Design review of the part built by this model. Coordinates are the model's own, in mm. A direction names the side the tool comes from. Coordinates: 2 decimals unless noted, no trailing zeros. Loops run counter-clockwise (first coordinate to the right, second up) from the corner with the lowest first, then second, coordinate; pieces in that order, holes last. Notation, with made-up numbers: (-15.5, -31) -> (43.5, -31) arc R21 ccw to (43.5, -19) -> close; hole circle Ø2 at (8, -4.75). An arc over 180 degrees is marked (long way). Answer as a JSON object with one key per item and string values.
Autodesk Inventor part; units mm, degrees
ref_plane "Work Plane1" through (-5.715, 0, 0) normal (1, 0, 0) x (0, 1, 0)
ref_plane "Work Plane2" through (-5.715, 0, 0) normal (1, 0, 0) x (0, 1, 0)
ref_plane "XZ Plane" through (0, 0, 0) normal (0, 1, 0) x (-1, 0, 0)
sketch "Sketch1" plane through (0, 0, 0) normal (0, 1, 0) x (-1, 0, 0)
  circle A0 centre (0, 0) radius 4.318
  circle A1 centre (0, 0) radius 5.715
  dimension "d0" = 8.636
  dimension "d1" = 11.43
extrude "Extrusion1" add sketch "Sketch1" along normal blind 3.302
sketch "Sketch2" plane through (0, 0, 0) normal (0, -1, 0) x (1, 0, 0)
  circle A0 centre (0, 0) radius 5.715
  circle A1 centre (0, 0) radius 1.8415
  dimension "d4" = 3.683
extrude "Extrusion2" add sketch "Sketch2" along normal blind 4.953
ref_plane "Work Plane1" through (-5.715, 0, 0) normal (1, 0, 0) x (0, 1, 0)
sketch "Sketch3" plane through (-5.715, 0, 0) normal (1, 0, 0) x (0, 1, 0)
  circle A0 centre (-2.54, 0) radius 1.651
  line L0 (-4.953, 5.715) -> (-4.953, -5.715)
  point P0 (0, 0)
  dimension "d7" = 3.302
  dimension "d8" = 2.413
extrude "Extrusion3" cut sketch "Sketch3" along normal blind 2.159
pattern_circular "Circular Pattern1" count 4 over 360 about axis through (0, 0, 0) along (0, 1, 0) of "Extrusion3"
ref_plane "Work Plane2" through (-5.715, 0, 0) normal (1, 0, 0) x (0, 1, 0)
sketch "Sketch4" plane through (-5.715, 0, 0) normal (1, 0, 0) x (0, 1, 0)
  circle A0 centre (2.032, 0) radius 1.524
  line L0 (3.302, -5.715) -> (3.302, 5.715)
  line L1 (2.032, -1.524) -> (3.302, -1.524)
  line L2 (2.032, 1.524) -> (3.302, 1.524)
  point P0 (0, 0)
  dimension "d14" = 3.048
  dimension "d15" = 1.27
extrude "Extrusion4" cut sketch "Sketch4" along normal blind 2.159 contours A0 L0 | L2 L0 A0 | A0 L0 L1 picked at (2.3744, -0.0612)
properties part number "SpoolCarrageMagnetMountREV2" material "ABS Plastic"
1) Clearance check with flat-ended pins moving along their axes: pin 1 Ø2.5 at (x, z) = (-1.5, 0) entering from +Y; pin 2 Ø1.5 at (x, y) = (-4.5, 2.5) entering from +Z; pin 3 Ø4 at (y, z) = (1, -4) entering from -X. State where each tip first meets the part, or that it passes through.
Completed:
{"pin 1": "y = 0", "pin 2": "z = 4.31", "pin 3": "x = -5.35"}
2) Add section B-B, the plane z = 0. Give the boundary of the cut face in (x, y) (1 decimal), and give its area (3 significant figures).
Completed:
{"outline": "(-5.7, -5) -> (-1.8, -5) -> (-1.8, 0) -> (-4.3, 0) -> (-4.3, 0.5) -> (-5.7, 0.5) -> (-5.7, -0.9) -> (-3.6, -0.9) -> (-3.6, -4.2) -> (-5.7, -4.2) -> close; (1.8, -5) -> (5.7, -5) -> (5.7, -4.2) -> (3.6, -4.2) -> (3.6, -0.9) -> (5.7, -0.9) -> (5.7, 3.3) -> (4.3, 3.3) -> (4.3, 0) -> (1.8, 0) -> close", "area": "29.4 mm²"}
3) Add section D-D, the plane y = -3.5. Give the boundary of the cut face in (x, z) (1 decimal).
Completed:
{"outline": "(-5.6, -1.3) arc R5.7 ccw to (-1.3, -5.6) -> (-1.3, -3.6) -> (1.3, -3.6) -> (1.3, -5.6) arc R5.7 ccw to (5.6, -1.3) -> (3.6, -1.3) -> (3.6, 1.3) -> (5.6, 1.3) arc R5.7 ccw to (1.3, 5.6) -> (1.3, 3.6) -> (-1.3, 3.6) -> (-1.3, 5.6) arc R5.7 ccw to (-5.6, 1.3) -> (-3.6, 1.3) -> (-3.6, -1.3) -> close; hole circle Ø3.7 at (0, 0)"}
4) Add section A-A, the plane x = 0. Give the boundary of the cut face in (y, z) (1 decimal).
Completed:
{"outline": "(-5, -5.7) -> (-4.2, -5.7) -> (-4.2, -3.6) -> (-0.9, -3.6) -> (-0.9, -5.7) -> (3.3, -5.7) -> (3.3, -4.3) -> (0, -4.3) -> (0, -1.8) -> (-5, -1.8) -> close; (-5, 1.8) -> (0, 1.8) -> (0, 4.3) -> (3.3, 4.3) -> (3.3, 5.7) -> (-0.9, 5.7) -> (-0.9, 3.6) -> (-4.2, 3.6) -> (-4.2, 5.7) -> (-5, 5.7) -> close"}
5) Add section C-C, the plane x = 4. Give the boundary of the cut face in (y, z), and give its area (3 significant figures).
Completed:
{"outline": "(-4.95, -4.08) -> (3.3, -4.08) -> (3.3, -1.63) -> (0, -1.63) -> (0, 1.63) -> (3.3, 1.63) -> (3.3, 4.08) -> (-4.95, 4.08) -> close; hole circle Ø3.3 at (-2.54, 0)", "area": "48.1 mm²"}
6) Wall thickness on probe 1 along Y at (x, z) = (0, 4.1); probe 2 along Z at (x, y) = (0, -2.7); probe 3 along Z at (x, y) = (0, 1) (3 decimals): over which ranges is each line inside the solid? List them lowest first.
Completed:
{"probe 1": "-4.95 to -4.19, -0.89 to 0", "probe 2": "-3.56 to -1.84, 1.84 to 3.56", "probe 3": "-5.715 to -4.318, 4.318 to 5.715"}
7) For faces 1 (the flat face through (-5, 3, 1.524)), 2 (the cylindrical face through (4.314, 1.628, -0.19)), 3 (the cylindrical face through (4.65, -2.9, -1.61)), list the 3-axis set-ups (+Z, -Z, +X, -X, +Y, -Y) from which the entire face can be reached by the end or side of a thin tool; tool diameter is ignored.
Completed:
{"face 1": "-X, +Y", "face 2": "+Y", "face 3": "+X"}
8) The part is to be moulded in two halves that separate along Y. For faces 4 (the cylindrical face through (0.85, -2.442, 1.634)), 5 (the cylindrical face through (-1.465, -1.778, -4.651)), 6 (the cylindrical face through (-4.89, 0.51, -0.03)), say which applies: pulls with the +Y half, pulls with the -Y half, needs draft (parallel to the pull), parting line crosses it, or undercut.
Completed:
{"face 4": "needs draft", "face 5": "undercut", "face 6": "pulls with the +Y half"}
